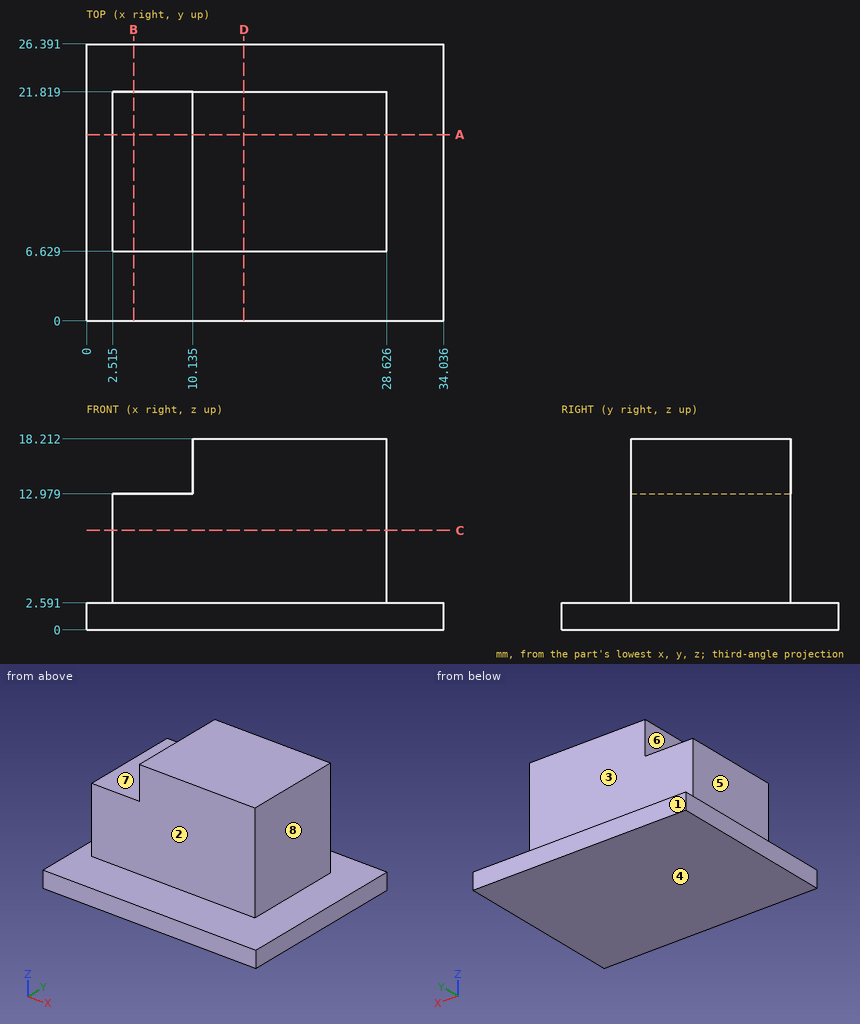
Could you check a few things on this drawing? It's one solid part, dimensions in mm from its lowest x, y, z. A direction names the side the tool comes from. Coordinates: 2 decimals unless noted, no trailing zeros. Order: outer loops, then holes, each group sorted by start corner. A loop starts at its lowest first (then second) coordinate and runs counter-clockwise, first axis right, second up. Notation, with made-up numbers: M -2,62.5 L 20,62.5 A6 ccw 20,67.5 Z; hole C -16.75,68.25 d11. An arc over 180 degrees is marked long. Use a Markdown table: item, result. Add a question column.
Q1. I want a section at D-D on x = 15. List the corners of the cut face in (y, z) for me.
Q2. If I drill on L1, parallel to X at y = 12, z = 12 (1 decimal); L2, parallel to X at y = 10, z = 16.5 (1 decimal); L3, parallel to Z at x = 16, y = 24, over which ranges is the centre line in solid material (lowest first)?
Q3. I want a section at A-A on y = 17.75. List the corners of the cut face in (x, z) for me (1 decimal), then the cut area to 3 significant figures.
Q4. I want a section at C-C on z = 9.5. List the corners of the cut face in (x, y) for me (1 decimal).
Q5. We'd pull the mould along X, two halves only. Please class the marked faces 6, 7 and 8: pulls with the +X half, pulls with the -X half, needs draft (parallel to the pull), parting line crosses it, or undercut.
Q6. Which directions (+Z, -Z, +X, -X, +Y, -Y) give clear straight access to the entire face, cutting with the end or side of a thin tool? Please do the marked faces 1, 2, 3, 4 and 5.
Q7. I want a section at B-B on x = 4.5. List the corners of the cut face in (y, z) for me.
Q8. I'm going to push flat-ended pins straight in: pin 1 (4 mm diameter, centred on x = 6, y = 13, fed in from +Z); pin 2 (6 mm diameter, centred on x = 27, y = 3, fed in from +Z); pin 3 (4.5 mm diameter, centred on x = 18.5, z = 8.5, fed in from +Y). Where does each tip first touch, or does it pass through?
Checked values:
| question | item | result |
|---|---|---|
| 1 | outline | M 0,0 L 26.39,0 L 26.39,2.59 L 21.82,2.59 L 21.82,18.21 L 6.63,18.21 L 6.63,2.59 L 0,2.59 Z |
| 2 | L1 | 2.5 to 28.6 |
| 2 | L2 | 10.1 to 28.6 |
| 2 | L3 | 0 to 2.59 |
| 3 | outline | M 0,0 L 34,0 L 34,2.6 L 28.6,2.6 L 28.6,18.2 L 10.1,18.2 L 10.1,13 L 2.5,13 L 2.5,2.6 L 0,2.6 Z |
| 3 | area | 456 mm² |
| 4 | outline | M 2.5,6.6 L 28.6,6.6 L 28.6,21.8 L 2.5,21.8 Z |
| 5 | face 6 | pulls with the -X half |
| 5 | face 7 | needs draft |
| 5 | face 8 | pulls with the +X half |
| 6 | face 1 | +Z, -Z, +X, -X, +Y |
| 6 | face 2 | +Z, +X, -X, -Y |
| 6 | face 3 | +Z, +X, -X, +Y |
| 6 | face 4 | -Z, +X, -X, +Y, -Y |
| 6 | face 5 | +Z, -X, +Y, -Y |
| 7 | outline | M 0,0 L 26.39,0 L 26.39,2.59 L 21.82,2.59 L 21.82,12.98 L 6.63,12.98 L 6.63,2.59 L 0,2.59 Z |
| 8 | pin 1 | z = 12.98 |
| 8 | pin 2 | z = 2.59 |
| 8 | pin 3 | y = 21.82 |
